Part model, mm, in its own coordinate system. A direction names the side the tool comes from. Give positions to 0.01 mm unless a question says otherwise; leave off trailing zeros. Order: outer loops, then holes, each group sorted by start corner. A loop starts at its lowest first (then second) coordinate and runs counter-clockwise, first axis right, second up.
1. Probe line 1 (Y direction, x = 140, z = 1.75) (3 decimals); line 2 (X direction, y = 26.5, z = 5.75); line 3 (X direction, y = 27, z = 1.5). List the from-to ranges inside material, lowest first.
2. Slice it at A-A on z = 4.75. List the corners of the cut face in (x, y) (3 decimals).
3. Which spindle directions (+Z, -Z, +X, -X, +Y, -Y) get a long thin tool onto all of the face, cutting with end or side? Do faces 1 (the flat face through (94, 0, 3)), 2 (the flat face through (219.377, 38.927, 3.131)), 3 (the flat face through (137, 15.875, 3)). Say none if no direction does.
4. Mould opens along X. For faces 4 (the flat face through (0, 26, 3)), 5 (the flat face through (29, 15.875, 3)), 6 (the flat face through (234.102, 6.159, 3.131)) say: +X half, -X half, draft (parallel to the pull), parting line (faces both ways), or undercut.
5. Slice it at D-D on y = 41. List the corners of the cut face in (x, z), and give its area (3 significant figures).
6. Slice it at B-B on y = 23.5. List the corners of the cut face in (x, z).
7. Drop flat-ended pins along their axis: pin 1 Ø1.9 at (x, z) = (129.5, 2) entering from -Y; pin 2 Ø1.5 at (y, z) = (12.5, 4.5) entering from +X; pin 3 Ø2 at (y, z) = (10.5, 4.5) entering from -X. Give the stop position or say it passes through.
8. Slice it at C-C on x = 174. List the corners of the cut face in (y, z).
from build123d import *

# Parameters (mm, degrees)
F1_DEPTH = 6.35


with BuildPart() as f1:
    # F0 (on Top) → F1 (new body)
    with BuildSketch(Plane.XY):
        with BuildLine():
            ThreePointArc((0, 12.7), (3.719744, 3.719744), (12.7, 0))
            Line((12.7, 0), (177.8, 0))
            Line((177.8, 0), (225.536385, -17.374623))
            Line((225.536385, -17.374623), (242.911008, 30.361762))
            Line((242.911008, 30.361762), (195.174623, 47.736385))
            ThreePointArc((195.174623, 47.736385), (186.621327, 50.028234), (177.8, 50.8))
            Line((177.8, 50.8), (12.7, 50.8))
            ThreePointArc((12.7, 50.8), (3.719744, 47.080256), (0, 38.1))
            Line((0, 38.1), (0, 12.7))
        make_face()
        with BuildLine():
            ThreePointArc((19.05, 15.875), (9.525, 25.4), (19.05, 34.925))
            Line((19.05, 34.925), (38.1, 34.925))
            ThreePointArc((38.1, 34.925), (47.625, 25.4), (38.1, 15.875))
            Line((38.1, 15.875), (19.05, 15.875))
        make_face(mode=Mode.SUBTRACT)
        with BuildLine():
            ThreePointArc((127, 15.875), (117.475, 25.4), (127, 34.925))
            Line((127, 34.925), (146.05, 34.925))
            ThreePointArc((146.05, 34.925), (155.575, 25.4), (146.05, 15.875))
            Line((146.05, 15.875), (127, 15.875))
        make_face(mode=Mode.SUBTRACT)
    extrude(amount=F1_DEPTH)


solid = f1.part
Data:
1. line 1: y = 0 to 15.875, 34.925 to 50.8
1. line 2: x = 0 to 9.59, 47.56 to 117.54, 155.51 to 241.51
1. line 3: x = 0 to 9.66, 47.49 to 117.61, 155.44 to 241.69
2. outline: (0, 12.7) arc R12.7 ccw to (12.7, 0) - (177.8, 0) - (225.536, -17.375) - (242.911, 30.362) - (195.175, 47.736) arc R50.8 ccw to (177.8, 50.8) - (12.7, 50.8) arc R12.7 ccw to (0, 38.1) - close; hole (19.05, 15.875) - (38.1, 15.875) arc R9.525 ccw to (38.1, 34.925) - (19.05, 34.925) arc R9.525 ccw to start; hole (127, 15.875) - (146.05, 15.875) arc R9.525 ccw to (146.05, 34.925) - (127, 34.925) arc R9.525 ccw to start
3. face 1: +Z, -Z, -X, -Y
3. face 2: +Z, -Z, +X, +Y
3. face 3: +Z, -Z
4. face 4: -X half
4. face 5: undercut
4. face 6: +X half
5. outline: (0.34, 0) - (213.68, 0) - (213.68, 6.35) - (0.34, 6.35) - close
5. area: 1,350 mm2
6. outline: (0, 0) - (9.72, 0) - (9.72, 6.35) - (0, 6.35) - close; (47.43, 0) - (117.67, 0) - (117.67, 6.35) - (47.43, 6.35) - close; (155.38, 0) - (240.41, 0) - (240.41, 6.35) - (155.38, 6.35) - close
7. pin 1: stops at y = 0
7. pin 2: stops at x = 236.68
7. pin 3: stops at x = 0.06
8. outline: (0, 0) - (50.8, 0) - (50.8, 6.35) - (0, 6.35) - close
